Build history of the part. All positions in model axes, mm. A direction names the side the tool comes from. Give positions to 0.01 mm unless a question says otherwise; leave off trailing zeros. Order: outer loops, then holes, each group sorted by start corner. A loop starts at its lowest first (then second) coordinate and runs counter-clockwise, first axis right, second up. Notation, with made-up numbers: (32.5, 44.25) - (76.5, 44.25) arc R33 ccw to (76.5, 79.25) - close; hole circle Ø4 at (65, 39.25). An arc over 180 degrees is marked (long way). Answer in a Markdown table with one row per item.
```python
from build123d import *

# Parameters (mm, degrees)
SKETCH1_R               = 1.905
BOSS_EXTRUDE1_DEPTH     = 7.62
CUT_EXTRUDE1_DEPTH      = 175.688488459
CUT_EXTRUDE2_DEPTH      = 176.172550646
BOSS_EXTRUDE3_DEPTH     = 6.35
SKETCH7_W               = 82.55
SKETCH7_H               = 25.4
BOSS_EXTRUDE4_DEPTH     = 7.62
CUT_EXTRUDE3_DEPTH      = 190.863938124
CUT_EXTRUDE3_DEPTH_BACK = 190.863938124
SKETCH8_R               = 1.905


with BuildPart() as part:
    # Sketch1 → Boss-Extrude1 (new body)
    with BuildSketch(Plane.XY):
        Polygon((-63.5, 0), (-50.8, 3.81), (50.8, 3.81), (63.5, 0), (50.8, -3.81), (10.16, -3.81), (10.16, -146.05), (6.35, -158.75), (2.54, -146.05), (2.54, -3.81), (-50.8, -3.81), align=None)
        with Locations((6.35, -85.09)):
            Circle(SKETCH1_R, mode=Mode.SUBTRACT)
    extrude(amount=-BOSS_EXTRUDE1_DEPTH)

    # Sketch3 → Cut-Extrude1 (cut, through all)
    with BuildSketch(Plane(origin=(0, 3.81, 0), x_dir=(1, 0, 0), z_dir=(0, 1, 0))):
        Polygon((-63.5, 0), (-50.8, 7.62), (-63.5, 7.62), align=None)
        Polygon((63.5, 7.62), (63.5, 0), (50.8, 7.62), align=None)
    extrude(amount=-CUT_EXTRUDE1_DEPTH, mode=Mode.SUBTRACT)

    # Sketch4 → Cut-Extrude2 (cut, through all)
    with BuildSketch(Plane(origin=(10.16, 0, 0), x_dir=(0, 0, -1), z_dir=(1, 0, 0))):
        Polygon((0, -158.75), (7.62, -146.05), (7.62, -158.75), align=None)
    extrude(amount=-CUT_EXTRUDE2_DEPTH, mode=Mode.SUBTRACT)

    # Sketch6 → Boss-Extrude3 (add)
    with BuildSketch(Plane.XY):
        Polygon((2.54, -146.05), (10.16, -146.05), (6.35, -158.75), align=None)
    extrude(amount=BOSS_EXTRUDE3_DEPTH)

    # Sketch7 → Boss-Extrude4 (add)
    with BuildSketch(Plane.ZY.offset(-2.54)):
        with Locations((-48.895, -88.9)):
            Rectangle(SKETCH7_W, SKETCH7_H)
    extrude(amount=-BOSS_EXTRUDE4_DEPTH)

    # Sketch8 → Cut-Extrude3 (cut, two sides: drawn at the far end of the back side and taken through both)
    with BuildSketch(Plane.XY.offset(-7.62).offset(-CUT_EXTRUDE3_DEPTH_BACK)):
        with Locations((6.35, -85.09)):
            Circle(SKETCH8_R)
    extrude(amount=CUT_EXTRUDE3_DEPTH + CUT_EXTRUDE3_DEPTH_BACK, mode=Mode.SUBTRACT)


solid = part.part
```
1. Cut at C-C on x = -35. Write the cut outline in (y, z).
Check result:
| item | result |
|---|---|
| outline | (-3.81, -7.62) - (3.81, -7.62) - (3.81, 0) - (-3.81, 0) - close |
2. Which spindle directions (+Z, -Z, +X, -X, +Y, -Y) get a long thin tool onto all of the face, cutting with end or side? Do faces 1 (the face through (6, -124, -7.62)), 2 (the face through (4, -15, -7.62)), 3 (the face through (-24, -3.81, -4)), 4 (the face through (10.16, -85, -32)), 5 (the face through (5, -49, 0)). Say none if no direction does.
Check result:
| item | result |
|---|---|
| face 1 | -Z, +X, -X, -Y |
| face 2 | -Z, +X, -X, +Y |
| face 3 | +Z, -Z, -X, -Y |
| face 4 | +Z, -Z, +X, -Y |
| face 5 | +Z, +X, -X, +Y |
3. Cut at A-A on y = -85.09. Write the cut outline in (x, z) (3 decimals), and give its area (3 significant figures).
Check result:
| item | result |
|---|---|
| outline | (2.54, -90.17) - (4.445, -90.17) - (4.445, 0) - (2.54, 0) - close; (8.255, -90.17) - (10.16, -90.17) - (10.16, 0) - (8.255, 0) - close |
| area | 344 mm² |
4. Probe line 1 (Y direction, x = 6.35, z = -25) (3 decimals); line 2 (X direction, y = -85.09, z = -24) (3 decimals); line 3 (X direction, y = -86.5, z = -39). List the from-to ranges inside material, lowest first.
Check result:
| item | result |
|---|---|
| line 1 | y = -101.6 to -86.995, -83.185 to -76.2 |
| line 2 | x = 2.54 to 4.445, 8.255 to 10.16 |
| line 3 | x = 2.54 to 5.07, 7.63 to 10.16 |
5. Cut at D-D on y = -65. Write the cut outline in (x, z), and give its area (3 significant figures).
Check result:
| item | result |
|---|---|
| outline | (2.54, -7.62) - (10.16, -7.62) - (10.16, 0) - (2.54, 0) - close |
| area | 58.1 mm² |
6. Cut at B-B on z = -12. Write the cut outline in (x, y) (3 decimals).
Check result:
| item | result |
|---|---|
| outline | (2.54, -101.6) - (10.16, -101.6) - (10.16, -76.2) - (2.54, -76.2) - close; hole circle Ø3.81 at (6.35, -85.09) |
7. Drop flat-ended pins along their axis: P1, Ø4, axis at x = 8, z = -55.5, coming from the -Y side; P2, Ø6, axis at x = 7, z = -48, coming from the +Y side; P3, Ø6, axis at x = -33, z = -5, coming from the -Y side. Give the stop position or say it passes through.
Check result:
| item | result |
|---|---|
| P1 | stops at y = -101.6 |
| P2 | stops at y = -76.2 |
| P3 | stops at y = -3.81 |
